from build123d import *

# Parameters (mm, degrees)
SKETCH2_R           = 25
BOSS_EXTRUDE1_DEPTH = 30
SKETCH3_R           = 27.5
BOSS_EXTRUDE2_DEPTH = 14


with BuildPart() as part:
    # Sketch1 → Revolve1 (revolve)
    with BuildSketch(Plane(origin=(0, 0, 0), x_dir=(0, 0, -1), z_dir=(1, 0, 0)), mode=Mode.PRIVATE) as revolve1_sk:
        with BuildLine():
            Line((-100, 0), (-100, 25))
            ThreePointArc((-100, 25), (0, 70.020961978), (100, 25))
            Line((100, 25), (100, 0))
            Line((100, 0), (-100, 0))
        make_face()
    revolve(revolve1_sk.sketch.rotate(Axis((0, 0, 74.117927805), (0, 0, -1)), 90), axis=Axis((0, 0, 74.117927805), (0, 0, -1)))

    # Sketch2 → Boss-Extrude1 (add)
    with BuildSketch(Plane.XY.offset(100)):
        Circle(SKETCH2_R)
    extrude(amount=BOSS_EXTRUDE1_DEPTH)

    # Sketch3 → Boss-Extrude2 (add)
    with BuildSketch(Plane(origin=(0, 0, -100), x_dir=(-1, 0, 0), z_dir=(0, 0, -1))):
        Circle(SKETCH3_R)
    extrude(amount=BOSS_EXTRUDE2_DEPTH)


solid = part.part
Model file for the job. Use its own axes, mm. A direction names the side the tool comes from. Round coordinates to 2 decimals unless told otherwise and drop trailing zeros. Order: outer loops, then holes, each group sorted by start corner. A loop starts at its lowest first (then second) coordinate and runs counter-clockwise, first axis right, second up.
(1) Band-saw the part on A-A (z = 115). List the corners of the cut face in (x, y).
(2) Pin check, flat tips, straight feed: pin 1 (2 mm diameter, centred on x = -42.5, y = -28, fed in from +Z); pin 2 (2 mm diameter, centred on x = 44.5, y = 24, fed in from +Z); pin 3 (10 mm diameter, centred on x = -47.5, y = -7, fed in from -Z). Stop position of each tip, or through.
(3) Pull direction Z, two halves, no side cores. Call faces 3 (the face through (0, 0, 130)), 4 (the face through (5.961, -26.846, -106.902)), 5 (the face through (-12.1, -22.3, -100)): released by +Z, released by -Z, zero draft, split by the parting line, or undercut.
(4) 3-axis set-ups, long thin cutter, end or side, ignore diameter. For faces 1 (the face through (23.846, 7.509, 114.79)), 2 (the face through (0, 0, -114)): which of +Z, -Z, +X, -X, +Y, -Y reach the whole face in a straight line?
(5) Drill centre lines: line 1 (Z direction, x = -25, y = -56); line 2 (Y direction, x = -51, z = -47.5); line 3 (Y direction, x = -34, z = 50). Where is each one in solid material? Low to high.
Verdict:
1. outline: circle Ø50 at (0, 0)
2. pin 1: stops at z = 70.51
2. pin 2: stops at z = 71.04
2. pin 3: stops at z = -80.53
3. face 3: released by +Z
3. face 4: zero draft
3. face 5: undercut
4. face 1: +Z
4. face 2: -Z, +X, -X, +Y, -Y
5. line 1: z = -47.4 to 47.4
5. line 2: y = -33.99 to 33.99
5. line 3: y = -49.81 to 49.81
